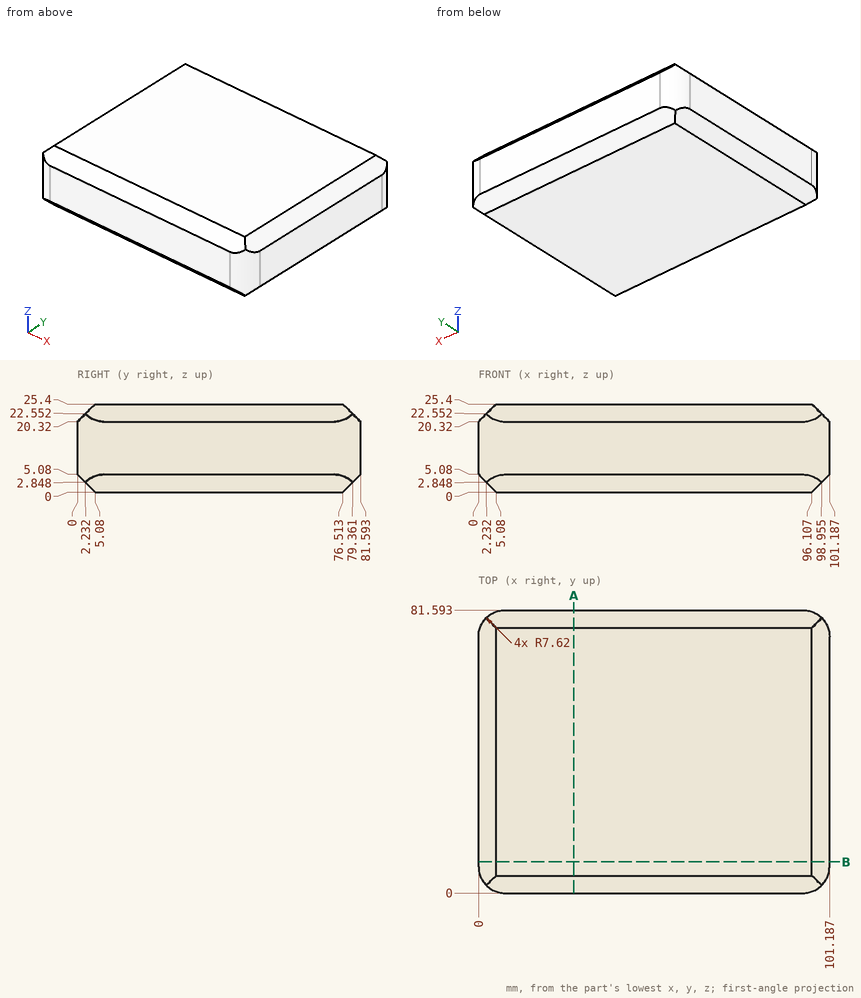
Source: three-view drawing plus pictorial views. Frame: mm from the lowest corner of the part. Round coordinates to 2 decimals unless told otherwise and drop trailing zeros. Loops run counter-clockwise (first coordinate to the right, second up) from the corner with the lowest first, then second, coordinate; pieces in that order, holes last.
Q1. Section B-B, the plane y = 9. Return loops of the section in (x, z), plus the area to 3 significant figures.
Q2. First-contact query: P1, Ø1.5, axis at y = 62.5, z = 21.5, coming from the +X side; P2, Ø1.5, axis at x = 90, z = 3, coming from the +Y side. Flat tips, straight axial feed; report the tip coordinate or a pass-through.
Q3. Section A-A, the plane x = 27.5. Return loops of the section in (y, z).
Q4. Ray query, line 1 (X direction, y = 32, z = 2.5); line 2 (X direction, y = 60, z = 24); line 3 (Y direction, x = 81, z = 2.5). Return the intervals inside material, ascending.
Solutions:
1. outline: (0, 5.08) - (5.08, 0) - (96.11, 0) - (101.19, 5.08) - (101.19, 20.32) - (96.11, 25.4) - (5.08, 25.4) - (0, 20.32) - close
1. area: 2,520 mm2
2. P1: stops at x = 100.76
2. P2: stops at y = 80.26
3. outline: (0, 5.08) - (5.08, 0) - (76.51, 0) - (81.59, 5.08) - (81.59, 20.32) - (76.51, 25.4) - (5.08, 25.4) - (0, 20.32) - close
4. line 1: x = 2.58 to 98.61
4. line 2: x = 3.68 to 97.51
4. line 3: y = 2.58 to 79.01
